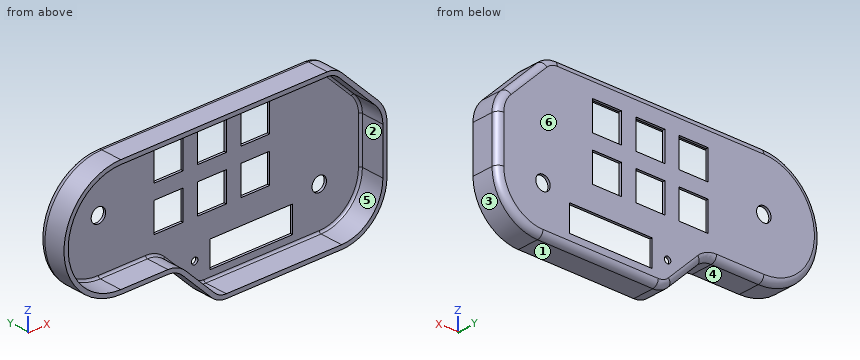
from build123d import *

# Parameters (mm, degrees)
SKETCH1_R           = 3.5
SKETCH1_W           = 14
SKETCH1_H           = 14
BOSS_EXTRUDE1_DEPTH = 1.2
FILLET1_R           = 10
BOSS_EXTRUDE2_DEPTH = 12
FILLET2_R           = 3
FILLET3_R           = 1
SKETCH4_R           = 1.5625
SKETCH4_W           = 40
SKETCH4_H           = 12.5
CUT_EXTRUDE1_DEPTH  = 171.515153338


with BuildPart() as part:
    # Sketch1 → Boss-Extrude1 (new body)
    with BuildSketch(Plane(origin=(0, 0, 0), x_dir=(1, 0, 0), z_dir=(0, 1, 0))):
        with BuildLine():
            Line((-125.065322034, 55), (-98.065322034, 55))
            Line((-98.065322034, 55), (-78.065322034, 75))
            Line((-78.065322034, 75), (-18.065322034, 75))
            ThreePointArc((-18.065322034, 75), (-2.508972848, 68.556349186), (3.934677966, 53))
            Line((3.934677966, 53), (3.934677966, 31))
            ThreePointArc((3.934677966, 31), (2.792870954, 25.259748515), (-0.458720316, 20.393398282))
            Line((-0.458720316, 20.393398282), (-20.852118598, 0))
            Line((-20.852118598, 0), (-25.734830863, 0))
            Line((-25.734830863, 0), (-125.065322034, 0))
            ThreePointArc((-125.065322034, 0), (-152.565322034, 27.5), (-125.065322034, 55))
        make_face()
        with Locations(Location((-125.065322034, 27.5, 0), (0, 0, 270))):
            Circle(SKETCH1_R, mode=Mode.SUBTRACT)
        with Locations(Location((-18.065322034, 53, 0), (0, 0, 270))):
            Circle(SKETCH1_R, mode=Mode.SUBTRACT)
        with Locations((-70.065322034, 17)):
            Rectangle(SKETCH1_W, SKETCH1_H, mode=Mode.SUBTRACT)
        with Locations((-91.065322034, 17)):
            Rectangle(SKETCH1_W, SKETCH1_H, mode=Mode.SUBTRACT)
        with Locations((-49.065322034, 17)):
            Rectangle(SKETCH1_W, SKETCH1_H, mode=Mode.SUBTRACT)
        with Locations((-70.065322034, 38)):
            Rectangle(SKETCH1_W, SKETCH1_H, mode=Mode.SUBTRACT)
        with Locations((-49.065322034, 38)):
            Rectangle(SKETCH1_W, SKETCH1_H, mode=Mode.SUBTRACT)
        with Locations((-91.065322034, 38)):
            Rectangle(SKETCH1_W, SKETCH1_H, mode=Mode.SUBTRACT)
    extrude(amount=BOSS_EXTRUDE1_DEPTH)

    # Fillet1
    fillet1_edges = [part.edges().sort_by_distance(p)[0] for p in [
        (-98.065322034, 0.6, -55),
        (-78.065322034, 0.6, -75),
        (-20.852118598, 0.6, 0),
    ]]
    fillet(fillet1_edges, radius=FILLET1_R)

    # Sketch3 → Boss-Extrude2 (add)
    with BuildSketch(Plane.XZ):
        with BuildLine():
            Line((-0.458720316, -20.393398282), (-17.92318641, -2.928932188))
            ThreePointArc((-17.92318641, -2.928932188), (-21.167419898, -0.761204675), (-24.994254222, 0))
            Line((-24.994254222, 0), (-125.065322034, 0))
            ThreePointArc((-125.065322034, 0), (-152.565322034, -27.5), (-125.065322034, -55))
            Line((-125.065322034, -55), (-102.207457658, -55))
            ThreePointArc((-102.207457658, -55), (-98.380623334, -55.761204675), (-95.136389846, -57.928932188))
            Line((-95.136389846, -57.928932188), (-80.994254222, -72.071067812))
            ThreePointArc((-80.994254222, -72.071067812), (-77.750020734, -74.238795325), (-73.92318641, -75))
            Line((-73.92318641, -75), (-18.065322034, -75))
            ThreePointArc((-18.065322034, -75), (-2.508972848, -68.556349186), (3.934677966, -53))
            Line((3.934677966, -53), (3.934677966, -31))
            ThreePointArc((3.934677966, -31), (2.792870954, -25.259748515), (-0.458720316, -20.393398282))
        make_face()
        with BuildLine():
            Line((-1.872933878, -21.807611845), (-19.337399973, -4.343145751))
            ThreePointArc((-19.337399973, -4.343145751), (-21.932786763, -2.60896374), (-24.994254222, -2))
            Line((-24.994254222, -2), (-125.065322034, -2))
            ThreePointArc((-125.065322034, -2), (-150.565322034, -27.5), (-125.065322034, -53))
            Line((-125.065322034, -53), (-102.207457658, -53))
            ThreePointArc((-102.207457658, -53), (-97.615256469, -53.91344561), (-93.722176283, -56.514718626))
            Line((-93.722176283, -56.514718626), (-79.58004066, -70.656854249))
            ThreePointArc((-79.58004066, -70.656854249), (-76.984653869, -72.39103626), (-73.92318641, -73))
            Line((-73.92318641, -73), (-18.065322034, -73))
            ThreePointArc((-18.065322034, -73), (-3.92318641, -67.142135624), (1.934677966, -53))
            Line((1.934677966, -53), (1.934677966, -31))
            ThreePointArc((1.934677966, -31), (0.945111889, -26.025115379), (-1.872933878, -21.807611845))
        make_face(mode=Mode.SUBTRACT)
    extrude(amount=BOSS_EXTRUDE2_DEPTH)

    # Fillet2
    fillet2_edges = [part.edges().sort_by_distance(p)[0] for p in [
        (-9.190953363, 1.2, -11.661165235),
        (-88.065322034, 1.2, -65),
        (-113.636389846, 1.2, -55),
        (-77.750020734, 1.2, -74.238795325),
        (-21.167419898, 1.2, -0.761204675),
        (-98.380623334, 1.2, -55.761204675),
        (2.792870954, 1.2, -25.259748515),
        (3.934677966, 1.2, -42),
        (-2.508972848, 1.2, -68.556349186),
        (-45.994254222, 1.2, -75),
        (-152.565322034, 1.2, -27.5),
        (-75.029788128, 1.2, 0),
    ]]
    fillet(fillet2_edges, radius=FILLET2_R)

    # Fillet3
    fillet3_edges = [part.edges().sort_by_distance(p)[0] for p in [
        (-97.615256469, 0, -53.91344561),
        (0.945111889, 0, -26.025115379),
        (-10.605166926, 0, -13.075378798),
        (-21.932786763, 0, -2.60896374),
        (-75.029788128, 0, -2),
        (-150.565322034, 0, -27.5),
        (-113.636389846, 0, -53),
        (-86.651108472, 0, -63.585786438),
        (-76.984653869, 0, -72.39103626),
        (-45.994254222, 0, -73),
        (-3.92318641, 0, -67.142135624),
        (1.934677966, 0, -42),
    ]]
    fillet(fillet3_edges, radius=FILLET3_R)

    # Sketch4 → Cut-Extrude1 (cut, through all)
    with BuildSketch(Plane(origin=(0, 1.2, 0), x_dir=(1, 0, 0), z_dir=(0, 1, 0))):
        with Locations(Location((-78.43359405, 62.814339828, 0), (0, 0, 270))):
            Circle(SKETCH4_R)
        with Locations((-50.92318641, 62.75)):
            Rectangle(SKETCH4_W, SKETCH4_H)
    extrude(amount=-CUT_EXTRUDE1_DEPTH, mode=Mode.SUBTRACT)


solid = part.part
Can you work these out from the model? Positions are in its coordinate system, mm. Face numbers are marked on the shaded views. A direction names the side the tool comes from. Coordinates: 2 decimals unless noted, no trailing zeros. Loops run counter-clockwise (first coordinate to the right, second up) from the corner with the lowest first, then second, coordinate; pieces in that order, holes last. Notation, with made-up numbers: M 15,-22.75 L 41,-22.75 A23 ccw 41,-6.75 Z; hole C 48,-20.75 d10. An arc over 180 degrees is marked long. Answer as CSV lines item,"result". Start each with the question number.
1. Suppose I cut it at A-A, the plane y = -9.5. List the corners of the cut face in (x, z) for me, plus the area to 3 significant figures.
2. For pin 1 Ø1.3 at (x, y) = (-54, 1) entering from -Z; pin 2 Ø1 at (y, z) = (0.5, -16) entering from +X; pin 3 Ø3 at (x, z) = (-45.5, -29) entering from -Y, each with a flat end and sliding along its axis, tell me the tip position at first contact or that it passes through.
3. If I drill on probe 1 along Z at (x, y) = (-59.5, -5); probe 2 along Z at (x, y) = (-124, -5); probe 3 along Y at (x, z) = (-73, -7), over which ranges is the centre line in solid material (lowest first)? Write a range as [from, to].
4. Suppose I cut it at B-B, the plane z = -16.5. Count the separate pieces of the cut face and the enclosed holes in it, plus the area to 3 significant figures.
5. Thinking about a two-plate mould opening in X: for the marked faces 1, 2 and 3, which applies, +X half, -X half, draft (parallel to the pull), parting line (faces both ways), or undercut?
6. For the marked faces 4, 5 and 6, which set-ups out of +Z, -Z, +X, -X, +Y, -Y let a thin tool reach every point of the face, with its end or its side?
Output:
1,outline,"M -125.07,-55 L -102.21,-55 A10 cw -95.14,-57.93 L -80.99,-72.07 A10 ccw -73.92,-75 L -18.07,-75 A22 ccw 3.93,-53 L 3.93,-31 A15 ccw -0.46,-20.39 L -17.92,-2.93 A10 ccw -24.99,0 L -125.07,0 A27.5 ccw Z; hole M -125.07,-53 L -102.21,-53 A12 cw -93.72,-56.51 L -79.58,-70.66 A8 ccw -73.92,-73 L -18.07,-73 A20 ccw 1.93,-53 L 1.93,-31 A13 ccw -1.87,-21.81 L -19.34,-4.34 A8 ccw -24.99,-2 L -125.07,-2 A25.5 ccw Z"
1,area,"791 mm^2"
2,pin 1,"stops at z = -74.09"
2,pin 2,"stops at x = -5.51"
2,pin 3,"stops at y = 0"
3,probe 1,"z = [-75, -73], [-2, 0]"
3,probe 2,"z = [-55, -53], [-2, 0]"
3,probe 3,"y = [0, 1.2]"
4,separate pieces,"4"
4,enclosed holes,"0"
4,area,"181 mm^2"
5,face 1,"draft"
5,face 2,"undercut"
5,face 3,"+X half"
6,face 4,"-Z, -X, +Y, -Y"
6,face 5,"-Y"
6,face 6,"+Z, -Z, +X, -X, +Y"
